Autodesk Inventor part; units mm, degrees
ref_plane "Work Plane1" through (-69.85, 17.4625, 0) normal (1, 0, 0) x (0, 0, -1)
ref_plane "YZ Plane" through (0, 0, 0) normal (1, 0, 0) x (0, 1, 0)
ref_plane "XZ Plane" through (0, 0, 0) normal (0, 1, 0) x (-1, 0, 0)
sketch "Sketch1" plane through (0, 0, 0) normal (0, 1, 0) x (-1, 0, 0)
  line L0 (0, 0) -> (139.7, 0)
  line L1 (139.7, 0) -> (139.7, -311.5225)
  line L2 (139.7, -311.5225) -> (0, -311.5225)
  line L3 (0, -311.5225) -> (0, 0)
  line L4 (4.7625, -4.7625) -> (134.9375, -4.7625)
  line L5 (134.9375, -4.7625) -> (134.9375, -106.3625)
  line L6 (134.9375, -106.3625) -> (4.7625, -106.3625)
  line L7 (4.7625, -106.3625) -> (4.7625, -4.7625)
  line L8 (121.977, -109.5375) -> (17.723, -109.5375)
  line L9 (17.723, -109.5375) -> (17.723, -305.1725)
  line L10 (17.723, -305.1725) -> (121.977, -305.1725)
  line L11 (121.977, -305.1725) -> (121.977, -109.5375)
  line L12 (128.327, -106.3625) -> (128.327, -311.5225)
  line L13 (11.373, -106.3625) -> (11.373, -311.5225)
  point P0 (69.85, -305.1725)
  point P1 (69.85, -311.5225)
  dimension "d0" = 139.7
  dimension "d1" = 311.5225
  dimension "d2" = 4.7625
  dimension "d3" = 4.7625
  dimension "d4" = 4.7625
  dimension "d5" = 101.6
  dimension "d6" = 104.254
  dimension "d7" = 6.35
  dimension "d8" = 195.635
  dimension "d9" = 6.35
  dimension "d10" = 6.35
extrude "Extrusion1" add sketch "Sketch1" along normal blind 29.175 contours L13 L6 L12 L2
extrude "Extrusion2" add sketch "Sketch1" along normal blind 4.7625 contours L11 L10 L9 L8
extrude "Extrusion3" add sketch "Sketch1" along normal blind 3.175 contours L6 L7 L4 L5
extrude "Extrusion4" add sketch "Sketch1" along normal blind 17.4625 contours L0 L1 L2 L12 L6 L5 L4 L7 L13 L3
sketch "Sketch2" plane through (-121.977, 29.175, -305.1725) normal (0, 0, 1) x (1, 0, 0)
  circle A0 centre (13.127, -13) radius 13
  circle A1 centre (39.127, -13) radius 13
  circle A2 centre (65.127, -13) radius 13
  circle A3 centre (91.127, -13) radius 13
  line L0 (-6.35, 0) -> (110.604, 0)
  point P0 (121.977, -29.175)
  point P1 (52.127, -13)
  point P2 (52.127, 0)
  dimension "d20" = 26
  dimension "d21" = 26
  dimension "d19" = 26
  dimension "d22" = 26
extrude "Extrusion5" cut sketch "Sketch2" along normal up to surface (195.635 mm away) contours A0 | A1 | A2 | A3
sketch "Sketch3" plane through (-17.723, 29.175, -109.5375) normal (0, 0, -1) x (-1, 0, 0)
  arc A0 (84.9017, -24.4125) -> (97.3523, -24.4125) centre (91.127, -13) ccw
  arc A1 (6.9017, -24.4125) -> (19.3523, -24.4125) centre (13.127, -13) ccw
  arc A2 (99.0645, -13) -> (83.1895, -13) centre (91.127, -13) ccw
  arc A3 (21.0645, -13) -> (5.1895, -13) centre (13.127, -13) ccw
  line L0 (97.3523, -24.4125) -> (104.254, -24.4125)
  line L1 (71.3523, -24.4125) -> (84.9017, -24.4125)
  line L2 (0, -24.4125) -> (6.9017, -24.4125)
  line L3 (19.3523, -24.4125) -> (32.9017, -24.4125)
  line L4 (99.0645, -13) -> (99.0645, -24.4125)
  line L5 (83.1895, -13) -> (83.1895, -24.4125)
  line L6 (21.0645, -13) -> (21.0645, -24.4125)
  line L7 (5.1895, -13) -> (5.1895, -24.4125)
  line L8 (99.0645, -24.4125) -> (83.1895, -24.4125)
  line L9 (-12.9605, -26) -> (117.2145, -26)
  line L10 (5.1895, -24.4125) -> (21.0645, -24.4125)
  point P0 (-17.723, -29.175)
  dimension "d25" = 15.875
  dimension "d26" = 15.875
extrude "Extrusion6" cut sketch "Sketch3" against normal up to surface (3.175 mm away) contours L1 L5 A2 L4 L0 L8 | L2 L7 A3 L6 L3 L10
sketch "Sketch5" plane through (0, 0, 0) normal (0, -1, 0) x (1, 0, 0)
  line L0 (12.7, 12.7) -> (-152.4, 12.7)
  line L1 (-152.4, 12.7) -> (-152.4, -324.2225)
  line L2 (-152.4, -324.2225) -> (12.7, -324.2225)
  line L3 (12.7, -324.2225) -> (12.7, 12.7)
  line L4 (0, 0) -> (0, -311.5225)
  line L5 (-139.7, 0) -> (0, 0)
  line L6 (-139.7, -311.5225) -> (-139.7, 0)
  line L7 (0, -311.5225) -> (-139.7, -311.5225)
  dimension "d32" = 12.7
  dimension "d33" = 12.7
  dimension "d34" = 12.7
  dimension "d35" = 12.7
extrude "Extrusion8" add sketch "Sketch5" against normal blind 3.175 contours L3 L2 L1 L0 | L4 L7 L6 L5
sketch "Sketch4" plane through (0, 3.175, 0) normal (0, 1, 0) x (1, 0, 0)
  line L0 (-4.7625, 4.7625) -> (-4.7625, 106.3625)
  line L1 (-4.7625, 106.3625) -> (-134.9375, 106.3625)
  line L2 (-134.9375, 106.3625) -> (-134.9375, 4.7625)
  line L3 (-134.9375, 4.7625) -> (-4.7625, 4.7625)
  line L4 (-134.9375, 4.7625) -> (-134.9375, 106.3625)
  line L5 (-134.9375, 30.1625) -> (-4.7625, 30.1625)
  line L6 (-4.7625, 4.7625) -> (-4.7625, 106.3625)
  line L7 (-134.9375, 30.1625) -> (-134.9375, 4.7625)
  line L8 (-4.7625, 4.7625) -> (-4.7625, 30.1625)
  line L9 (-4.7625, 4.7625) -> (-134.9375, 4.7625)
  line L10 (-134.9375, 4.7625) -> (-4.7625, 4.7625)
  point P0 (0, 0)
  dimension "d29" = 25.4
extrude "Extrusion7" cut sketch "Sketch4" against normal blind 17.4625 contours L3 L2 L5 L0
ref_plane "Work Plane1" through (-69.85, 17.4625, 0) normal (1, 0, 0) x (0, 0, -1)
equation "\"d0\" = width"
equation "\"d1\" = length"
equation "\"d8\" = battery_length"
equation "\"d11\" = height"
equation "\"d13\" = bottom_thickness"
equation "\"width\" = 139.7"
equation "\"bottom_thickness\" = 4.7625"
equation "\"battery_length\" = 195.635"
properties part number "BatteryBox" material "ABS Plastic"
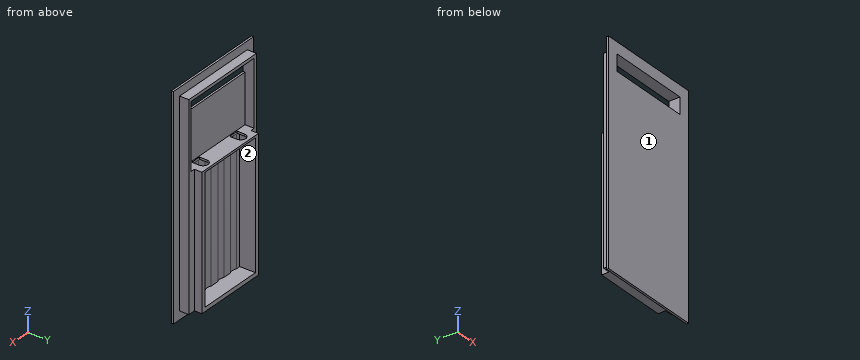
Geometry check sheet. Reference: the model listing, model coordinates, mm. Face numbers are marked on the shaded views. Give positions to 0.01 mm unless a question says otherwise; leave off trailing zeros. Write each loop counter-clockwise with the first axis right and the second up, starting at its lowest first coordinate (ties: lowest second). Pieces come first, ordered by that corner, then holes. Notation, with made-up numbers: (65.5, -22.5) - (75.5, -22.5) arc R17 cw to (75.5, 10.5) - close; hole circle Ø6 at (44, -21). An arc over 180 degrees is marked (long way). Put each result on its own line as item: value.
1. Thickness scan on line 1 (Z direction, x = -43.5, y = 11.25); line 2 (X direction, y = 11.75, z = -64.5); line 3 (X direction, y = 20, z = -224). Record the ranges inside material, lowest first.
Ans:
line 1: z = -311.52 to -305.17, -109.54 to -106.36, -4.76 to 0
line 2: x = -139.7 to -134.94, -4.76 to 0
line 3: x = -128.33 to -121.98, -17.72 to -11.37
2. Go/stop test with flat-tipped pins: pin 1 (3.5 mm diameter, centred on y = 12, z = -107.5, fed in from -X); pin 2 (4.5 mm diameter, centred on x = -87.5, y = 8, fed in from +Z); pin 3 (1 mm diameter, centred on y = 9, z = -85.5, fed in from +X). Record where each tip stops, or that it passes through.
Ans:
pin 1: stops at x = -139.7
pin 2: stops at z = 0
pin 3: stops at x = 0
3. Sectioned sample at A-A, the plane x = -131.5. Enter the section's corners in (y, z) (1 decimal).
Ans:
outline: (0, -324.2) - (3.2, -324.2) - (3.2, -311.5) - (17.5, -311.5) - (17.5, -106.4) - (3.2, -106.4) - (3.2, -30.2) - (0, -30.2) - close; (0, -4.8) - (17.5, -4.8) - (17.5, 0) - (3.2, 0) - (3.2, 12.7) - (0, 12.7) - close
4. Draft check along X on the marked faces 1 and 2. Enter one of: +X half, -X half, draft (parallel to the pull), parting line (faces both ways), or undercut.
Ans:
face 1: draft
face 2: undercut
5. Sectioned sample at B-B, the plane y = 9.75. Enter the section's corners in (x, z), plus the area to 3 significant figures.
Ans:
outline: (-139.7, -311.52) - (0, -311.52) - (0, 0) - (-139.7, 0) - close; (-100.91, -109.54) - (-38.79, -109.54) - (-38.79, -106.36) - (-100.91, -106.36) - close; hole (-134.94, -106.36) - (-116.79, -106.36) - (-116.79, -109.54) - (-121.98, -109.54) - (-121.98, -305.17) - (-17.72, -305.17) - (-17.72, -109.54) - (-22.91, -109.54) - (-22.91, -106.36) - (-4.76, -106.36) - (-4.76, -4.76) - (-134.94, -4.76) - close
area: 9,800 mm²
6. Sectioned sample at C-C, the plane x = -30.85. Enter the section's corners in (y, z) (1 decimal), plus the area to 3 significant figures.
Ans:
outline: (0, -324.2) - (3.2, -324.2) - (3.2, -311.5) - (29.2, -311.5) - (29.2, -305.2) - (3.2, -305.2) - (3.2, -109.5) - (4.8, -109.5) - (4.8, -106.4) - (3.2, -106.4) - (3.2, -30.2) - (0, -30.2) - close; (0, -4.8) - (17.5, -4.8) - (17.5, 0) - (3.2, 0) - (3.2, 12.7) - (0, 12.7) - close; (24.1, -109.5) - (29.2, -109.5) - (29.2, -106.4) - (24.1, -106.4) - close
area: 1,240 mm²
